from build123d import *

# Parameters (mm, degrees)
SKETCH1_R           = 1.5
SKETCH1_R_2         = 1
BOSS_EXTRUDE1_DEPTH = 3.175


with BuildPart() as part:
    # Sketch1 → Boss-Extrude1 (new body)
    with BuildSketch(Plane.XY):
        Polygon((6.35, 12.7), (6.35, 9.525), (12.7, 9.525), (12.7, 12.7), (19.05, 12.7), (19.05, 0), (0, 0), (0, 12.7), align=None)
        with Locations((12.7, 5.08)):
            Circle(SKETCH1_R, mode=Mode.SUBTRACT)
        with Locations((6.35, 5.08)):
            Circle(SKETCH1_R_2, mode=Mode.SUBTRACT)
    extrude(amount=BOSS_EXTRUDE1_DEPTH)


solid = part.part
Check sheet for the modelled part. Datum: model origin and axes. Units: mm. A direction names the side the tool comes from. Give positions to 0.01 mm unless a question says otherwise; leave off trailing zeros. Order: outer loops, then holes, each group sorted by start corner. A loop starts at its lowest first (then second) coordinate and runs counter-clockwise, first axis right, second up. Notation, with made-up numbers: M -17,24 L 22,24 A22 ccw 22,40 Z; hole C -22,-13.75 d1. An arc over 180 degrees is marked long. Answer as CSV lines item,"result". Start each with the question number.
Item 1: Cross-section at A-A on y = 5.08. Enter the section's corners in (x, z) (3 decimals), plus the area to 3 significant figures.
Item 2: Cross-section at D-D on x = 13.5. Enter the section's corners in (y, z) (3 decimals), plus the area to 3 significant figures.
Item 3: Thickness scan on line 1 (X direction, y = 10.5, z = 1.3); line 2 (Y direction, x = 12.75, z = 3); line 3 (X direction, y = 4.5, z = 2). Record the ranges inside material, lowest first. Write a range as [from, to].
Item 4: Cross-section at C-C on z = 0.65. Enter the section's corners in (x, y) (3 decimals), plus the area to 3 significant figures.
Item 5: Mould release check, pull along Y, two halves, no side actions. Record for faces 3 (the face through (10, 0, 2)), 4 (the face through (19.05, 6, 2)), 5 (the face through (3, 12.7, 2)), 6 (the face through (13.39, 3.75, 1.57)): +Y half, -Y half, draft (parallel to the pull), parting line (faces both ways), or undercut.
Item 6: Tool access check on faces 1 (the face through (9, 9.525, 2)), 2 (the face through (10, 6, 0)). Record the directions out of +Z, -Z, +X, -X, +Y, -Y that give a thin tool (end or side, any length) a straight path to the whole face; none if there is none.
Item 7: Gauge pin test, flat end, axial feed: P1, Ø1.6, axis at x = 9, z = 1.5, coming from the +Y side (3 decimals). Record the tip position at first contact, or that the pin passes through.
Item 8: Cross-section at B-B on x = 7. Enter the section's corners in (y, z) (3 decimals).
Established:
1,outline,"M 0,0 L 5.35,0 L 5.35,3.175 L 0,3.175 Z; M 7.35,0 L 11.2,0 L 11.2,3.175 L 7.35,3.175 Z; M 14.2,0 L 19.05,0 L 19.05,3.175 L 14.2,3.175 Z"
1,area,"44.6 mm^2"
2,outline,"M 0,0 L 3.811,0 L 3.811,3.175 L 0,3.175 Z; M 6.349,0 L 12.7,0 L 12.7,3.175 L 6.349,3.175 Z"
2,area,"32.3 mm^2"
3,line 1,"x = [0, 6.35], [12.7, 19.05]"
3,line 2,"y = [0, 3.58], [6.58, 12.7]"
3,line 3,"x = [0, 5.54], [7.16, 11.32], [14.08, 19.05]"
4,outline,"M 0,0 L 19.05,0 L 19.05,12.7 L 12.7,12.7 L 12.7,9.525 L 6.35,9.525 L 6.35,12.7 L 0,12.7 Z; hole C 6.35,5.08 d2; hole C 12.7,5.08 d3"
4,area,"212 mm^2"
5,face 3,"-Y half"
5,face 4,"draft"
5,face 5,"+Y half"
5,face 6,"undercut"
6,face 1,"+Z, -Z, +Y"
6,face 2,"-Z, +X, -X, +Y, -Y"
7,P1,"stops at y = 9.525"
8,outline,"M 0,0 L 4.32,0 L 4.32,3.175 L 0,3.175 Z; M 5.84,0 L 9.525,0 L 9.525,3.175 L 5.84,3.175 Z"
